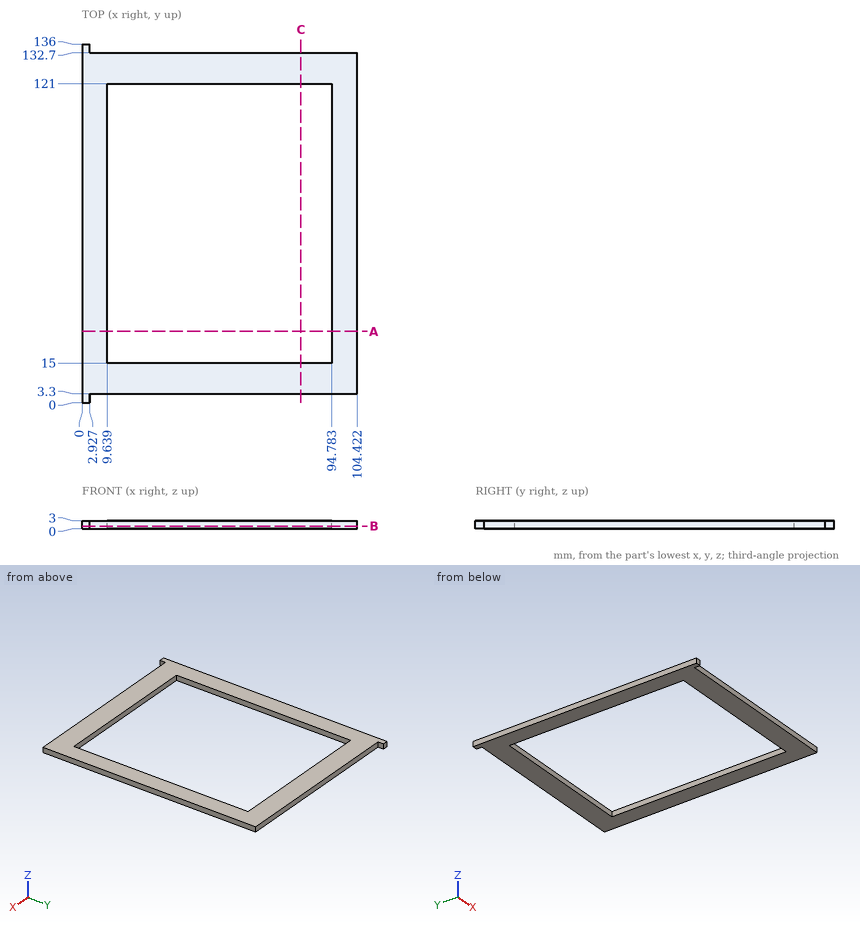
The drawing under review shows one solid part. Ordinate dimensions are in mm from its lowest x, y, z. Coordinates: 2 decimals unless noted, no trailing zeros. Loops run counter-clockwise (first coordinate to the right, second up) from the corner with the lowest first, then second, coordinate; pieces in that order, holes last. Notation, with made-up numbers: (59, -31.75) -> (80, -31.75) arc R14 ccw to (80, -26.75) -> close; hole circle Ø4 at (66.25, 32). An arc over 180 degrees is marked (long way). Answer as a JSON object with one key per item and string values.
Q1. Take a section at A-A on y = 27. Give the boundary of the cut face in (x, z).
Answer block:
{"outline": "(0, 0) -> (9.64, 0) -> (9.64, 3) -> (0, 3) -> close; (94.78, 0) -> (104.42, 0) -> (104.42, 3) -> (94.78, 3) -> close"}
Q2. Clearance check with flat-ended pins moving along their axes: pin 1 Ø0.9 at (x, z) = (34.5, 1.5) entering from -Y; pin 2 Ø0.9 at (x, z) = (69.5, 1.5) entering from +Y; pin 3 Ø0.9 at (y, z) = (134.5, 2) entering from +X. State where each tip first meets the part, or that it passes through.
Answer block:
{"pin 1": "stops at y = 3.3", "pin 2": "stops at y = 132.7", "pin 3": "stops at x = 2.93"}
Q3. To check wall thickness, follow L1, parallel to X at y = 108, z = 0.1; L2, parallel to Y at x = 23, z = 0.65; L3, parallel to Y at x = 99, z = 0.4. State the ranges of each line that lie inside material, in increasing order.
Answer block:
{"L1": "x = 0 to 9.64, 94.78 to 104.42", "L2": "y = 3.3 to 15, 121 to 132.7", "L3": "y = 3.3 to 132.7"}
Q4. Take a section at C-C on x = 83. Give the boundary of the cut face in (y, z).
Answer block:
{"outline": "(3.3, 0) -> (15, 0) -> (15, 3) -> (3.3, 3) -> close; (121, 0) -> (132.7, 0) -> (132.7, 3) -> (121, 3) -> close"}
Q5. Take a section at B-B on z = 0.95. Give the boundary of the cut face in (x, y), plus the area to 3 significant figures.
Answer block:
{"outline": "(0, 0) -> (2.93, 0) -> (2.93, 3.3) -> (104.42, 3.3) -> (104.42, 132.7) -> (2.93, 132.7) -> (2.93, 136) -> (0, 136) -> close; hole (9.64, 15) -> (94.78, 15) -> (94.78, 121) -> (9.64, 121) -> close", "area": "4,510 mm^2"}
